```python
from build123d import *

# Parameters (mm, degrees)
F0_W     = 101.0093018413
F0_H     = 101.0093018413
F1_DEPTH = 5.08
F2_W     = 101.0093018413
F2_H     = 101.0093018413
F2_W_2   = 92.3733018413
F2_H_2   = 92.3733018413
F3_DEPTH = 2.54


# Not quite as in the source:
# - the program builds the solid bodies; features that only make, move or delete a surface that nothing else refers to are left out


with BuildPart() as f1:
    # F0 (on Front) → F1 (new body)
    with BuildSketch(Plane.XZ):
        Rectangle(F0_W, F0_H)
    extrude(amount=F1_DEPTH)

    # F2 (on face) → F3 (join)
    with BuildSketch(Plane.XZ.offset(5.08)):
        Rectangle(F2_W, F2_H)
        Rectangle(F2_W_2, F2_H_2, mode=Mode.SUBTRACT)
    extrude(amount=F3_DEPTH)


solid = f1.part
```
Check sheet for the modelled part. Datum: model origin and axes. Units: mm. A direction names the side the tool comes from. Round coordinates to 2 decimals unless told otherwise and drop trailing zeros. Order: outer loops, then holes, each group sorted by start corner. A loop starts at its lowest first (then second) coordinate and runs counter-clockwise, first axis right, second up. Notation, with made-up numbers: (76.25, 8.5) - (110.25, 8.5) arc R32 ccw to (110.25, 46.5) - close; hole circle Ø1 at (0, 40). An arc over 180 degrees is marked (long way). Answer as CSV lines item,"result". Start each with the question number.
1) Depth check by flat-ended pin: pin 1 (6 mm diameter, centred on x = 7.5, z = 40, fed in from +Y); pin 2 (5 mm diameter, centred on x = -17.5, z = -7.5, fed in from -Y). Enter the tip coordinate at first touch or a pass-through.
2) Tool access check on faces 1 (the face through (-1, -6, 46.187)), 2 (the face through (-50.505, -4, -1)). Record the directions out of +Z, -Z, +X, -X, +Y, -Y that give a thin tool (end or side, any length) a straight path to the whole face; none if there is none.
3) Section check C-C (z = -26). Record the cut outline in (x, y), then the cut area to 3 significant figures.
4) Scan lines: probe 1 along Z at (x, y) = (-23, -6.25); probe 2 along Y at (x, z) = (-3, -21). Record each from-to range of solid material in increasing order.
5) Section check B-B (x = 29). Record the cut outline in (y, z).
6) Section check A-A (y = -6.25). Record the cut outline in (x, z), then the cut area to 3 significant figures.
7) Draft check along Z on faces 3 (the face through (-1, -4, 50.505)), 4 (the face through (-1, -4, -50.505)), 5 (the face through (50.505, -4, -1)), 6 (the face through (46.187, -6, -1)). Enter one of: +Z half, -Z half, draft (parallel to the pull), parting line (faces both ways), or undercut.
Determined:
1,pin 1,"y = 0"
1,pin 2,"y = -5.08"
2,face 1,"-Y"
2,face 2,"+Z, -Z, -X, +Y, -Y"
3,outline,"(-50.5, -7.62) - (-46.19, -7.62) - (-46.19, -5.08) - (46.19, -5.08) - (46.19, -7.62) - (50.5, -7.62) - (50.5, 0) - (-50.5, 0) - close"
3,area,"535 mm^2"
4,probe 1,"-50.5 to -46.19, 46.19 to 50.5"
4,probe 2,"-5.08 to 0"
5,outline,"(-7.62, -50.5) - (0, -50.5) - (0, 50.5) - (-7.62, 50.5) - (-7.62, 46.19) - (-5.08, 46.19) - (-5.08, -46.19) - (-7.62, -46.19) - close"
6,outline,"(-50.5, -50.5) - (50.5, -50.5) - (50.5, 50.5) - (-50.5, 50.5) - close; hole (-46.19, -46.19) - (46.19, -46.19) - (46.19, 46.19) - (-46.19, 46.19) - close"
6,area,"1,670 mm^2"
7,face 3,"+Z half"
7,face 4,"-Z half"
7,face 5,"draft"
7,face 6,"undercut"
